Build history of the part. All positions in model axes, mm. A direction names the side the tool comes from. Coordinates: 2 decimals unless noted, no trailing zeros. Order: outer loops, then holes, each group sorted by start corner. A loop starts at its lowest first (then second) coordinate and runs counter-clockwise, first axis right, second up. Notation, with made-up numbers: (-34.75, 45) - (-9.75, 45) arc R19 ccw to (-9.75, 82) - close; hole circle Ø5 at (81.5, 9). An arc over 180 degrees is marked (long way). Write each question's results on one line, items separated by ' | '.
from build123d import *

# Parameters (mm, degrees)
SKETCH_1_W          = 71
SKETCH_1_H          = 46
SKETCH_1_W_2        = 68
SKETCH_1_H_2        = 43
EXTRUDE_1_DEPTH     = 15
SKETCH_2_R          = 2
SKETCH_2_W          = 71
SKETCH_2_H          = 46
EXTRUDE_2_DEPTH     = 2
EXTRUDE_START       = 2
SKETCH_2_2_R        = 2
SKETCH_2_2_W        = 71
SKETCH_2_2_H        = 46
EXTRUDE_3_DEPTH     = 2
SKETCH_3_R          = 2
CUT_EXTRUDE_1_DEPTH = 96.766643462


with BuildPart() as part:
    # Sketch 1 → Extrude 1 (new body)
    with BuildSketch(Plane(origin=(0, 0, 0), x_dir=(1, 0, 0), z_dir=(0, 1, 0))):
        with Locations((34, 21.5)):
            Rectangle(SKETCH_1_W, SKETCH_1_H)
        with Locations((34, 21.5)):
            Rectangle(SKETCH_1_W_2, SKETCH_1_H_2, mode=Mode.SUBTRACT)
    extrude(amount=EXTRUDE_1_DEPTH)

    # Sketch 2 → Extrude 2 (add)
    with BuildSketch(Plane.XZ):
        with BuildLine():
            Line((76.5, -46.5), (-8.5, -46.5))
            ThreePointArc((-8.5, -46.5), (-12.035533906, -45.035533906), (-13.5, -41.5))
            Line((-13.5, -41.5), (-13.5, -1.5))
            ThreePointArc((-13.5, -1.5), (-12.035533906, 2.035533906), (-8.5, 3.5))
            Line((-8.5, 3.5), (76.5, 3.5))
            ThreePointArc((76.5, 3.5), (80.035533906, 2.035533906), (81.5, -1.5))
            Line((81.5, -1.5), (81.5, -41.5))
            ThreePointArc((81.5, -41.5), (80.035533906, -45.035533906), (76.5, -46.5))
        make_face()
        with Locations(Location((76, -41.5, 0), (0, 0, 270))):
            Circle(SKETCH_2_R, mode=Mode.SUBTRACT)
        with Locations(Location((76, -1.5, 0), (0, 0, 90))):
            Circle(SKETCH_2_R, mode=Mode.SUBTRACT)
        with Locations(Location((-8, -1.5, 0), (0, 0, 270))):
            Circle(SKETCH_2_R, mode=Mode.SUBTRACT)
        with Locations(Location((-8, -41.5, 0), (0, 0, 90))):
            Circle(SKETCH_2_R, mode=Mode.SUBTRACT)
        with Locations((34, -21.5)):
            Rectangle(SKETCH_2_W, SKETCH_2_H, mode=Mode.SUBTRACT)
    extrude(amount=-EXTRUDE_2_DEPTH)

    # Sketch 2_2 → Extrude 3 (add)
    with BuildSketch(Plane.XZ.offset(EXTRUDE_START)):
        with BuildLine():
            Line((76.5, -46.5), (-8.5, -46.5))
            ThreePointArc((-8.5, -46.5), (-12.035533906, -45.035533906), (-13.5, -41.5))
            Line((-13.5, -41.5), (-13.5, -1.5))
            ThreePointArc((-13.5, -1.5), (-12.035533906, 2.035533906), (-8.5, 3.5))
            Line((-8.5, 3.5), (76.5, 3.5))
            ThreePointArc((76.5, 3.5), (80.035533906, 2.035533906), (81.5, -1.5))
            Line((81.5, -1.5), (81.5, -41.5))
            ThreePointArc((81.5, -41.5), (80.035533906, -45.035533906), (76.5, -46.5))
        make_face()
        with Locations(Location((76, -41.5, 0), (0, 0, 270))):
            Circle(SKETCH_2_2_R, mode=Mode.SUBTRACT)
        with Locations(Location((76, -1.5, 0), (0, 0, 90))):
            Circle(SKETCH_2_2_R, mode=Mode.SUBTRACT)
        with Locations(Location((-8, -1.5, 0), (0, 0, 270))):
            Circle(SKETCH_2_2_R, mode=Mode.SUBTRACT)
        with Locations(Location((-8, -41.5, 0), (0, 0, 90))):
            Circle(SKETCH_2_2_R, mode=Mode.SUBTRACT)
        with Locations((34, -21.5)):
            Rectangle(SKETCH_2_2_W, SKETCH_2_2_H, mode=Mode.SUBTRACT)
    extrude(amount=-EXTRUDE_3_DEPTH)

    # Sketch 3 → Cut-Extrude 1 (cut, through all)
    with BuildSketch(Plane.XY.offset(1.5)):
        with Locations((34, 8.5)):
            Circle(SKETCH_3_R)
    extrude(amount=-CUT_EXTRUDE_1_DEPTH, mode=Mode.SUBTRACT)


solid = part.part
1. Two-plate mould, pull along Y, no slides. Class faces 4 (the face through (-9.352, -0.028, -42.974)), 5 (the face through (35.908, 9.101, 0.76)), 6 (the face through (31, 2, -45)), 7 (the face through (31, -2, -45)): +Y half, -Y half, draft (parallel to the pull), parting line (faces both ways), or undercut.
Solved:
face 4: draft | face 5: undercut | face 6: +Y half | face 7: -Y half
2. Band-saw the part on D-D on y = 1. Give the cut face in (x, z).
Solved:
outline: (-13.5, -41.5) arc R5 ccw to (-8.5, -46.5) - (76.5, -46.5) arc R5 ccw to (81.5, -41.5) - (81.5, -1.5) arc R5 ccw to (76.5, 3.5) - (-8.5, 3.5) arc R5 ccw to (-13.5, -1.5) - close; hole circle Ø4 at (-8, -41.5); hole circle Ø4 at (-8, -1.5); hole (0, -43) - (68, -43) - (68, 0) - (0, 0) - close; hole circle Ø4 at (76, -41.5); hole circle Ø4 at (76, -1.5)
3. Band-saw the part on A-A on y = 5.5. Give the cut face in (x, z), then the cut area to 3 significant figures.
Solved:
outline: (-1.5, -44.5) - (69.5, -44.5) - (69.5, 1.5) - (-1.5, 1.5) - close; hole (0, -43) - (68, -43) - (68, 0) - (0, 0) - close | area: 342 mm2
4. Band-saw the part on B-B on x = 34. Give the cut face in (y, z).
Solved:
outline: (-2, -46.5) - (2, -46.5) - (2, -44.5) - (6.5, -44.5) - (6.5, -43) - (0, -43) - (0, -44.5) - (-2, -44.5) - close; (-2, 1.5) - (0, 1.5) - (0, 0) - (6.5, 0) - (6.5, 1.5) - (2, 1.5) - (2, 3.5) - (-2, 3.5) - close; (10.5, -44.5) - (15, -44.5) - (15, -43) - (10.5, -43) - close; (10.5, 0) - (15, 0) - (15, 1.5) - (10.5, 1.5) - close
5. Band-saw the part on C-C on z = -28.5. Give the cut face in (x, y), then the cut area to 3 significant figures.
Solved:
outline: (-13.5, -2) - (-1.5, -2) - (-1.5, 0) - (0, 0) - (0, 15) - (-1.5, 15) - (-1.5, 2) - (-13.5, 2) - close; (68, 0) - (69.5, 0) - (69.5, -2) - (81.5, -2) - (81.5, 2) - (69.5, 2) - (69.5, 15) - (68, 15) - close | area: 141 mm2
6. Probe line 1 (X direction, y = -0.8, z = -41.5); line 2 (X direction, y = 0.9, z = -41.5); line 3 (X direction, y = 7.75, z = -14). List the from-to ranges inside material, lowest first.
Solved:
line 1: x = -13.5 to -10, -6 to -1.5, 69.5 to 74, 78 to 81.5 | line 2: x = -13.5 to -10, -6 to 0, 68 to 74, 78 to 81.5 | line 3: x = -1.5 to 0, 68 to 69.5
7. Drop flat-ended pins along their axis: pin 1 Ø2 at (x, y) = (28, 7.5) entering from +Z; pin 2 Ø8 at (y, z) = (8.5, -38) entering from +X; pin 3 Ø3 at (x, z) = (-8, -1.5) entering from -Y; pin 4 Ø3 at (y, z) = (7.5, -8) entering from -X. Give the stop position or say it passes through.
Solved:
pin 1: stops at z = 1.5 | pin 2: stops at x = 69.5 | pin 3: passes through | pin 4: stops at x = -1.5
8. Tool access for faces 1 (the face through (68, 7, -21)), 2 (the face through (69.5, 8, -21)), 3 (the face through (-1.5, -1, -22)): list every direction of +Z, -Z, +X, -X, +Y, -Y with a clear straight run to the whole face (end or side of a thin tool).
Solved:
face 1: +Y, -Y | face 2: +Z, -Z, +X, +Y | face 3: -Y
